Answer from the drawing. Dimensions are ordinates in mm from the lowest x, y and z of the part. A direction names the side the tool comes from. Give positions to 0.01 mm unless a question says otherwise; leave off trailing zeros. Order: outer loops, then holes, each group sorted by start corner. A loop starts at its lowest first (then second) coordinate and runs counter-clockwise, first axis right, second up.
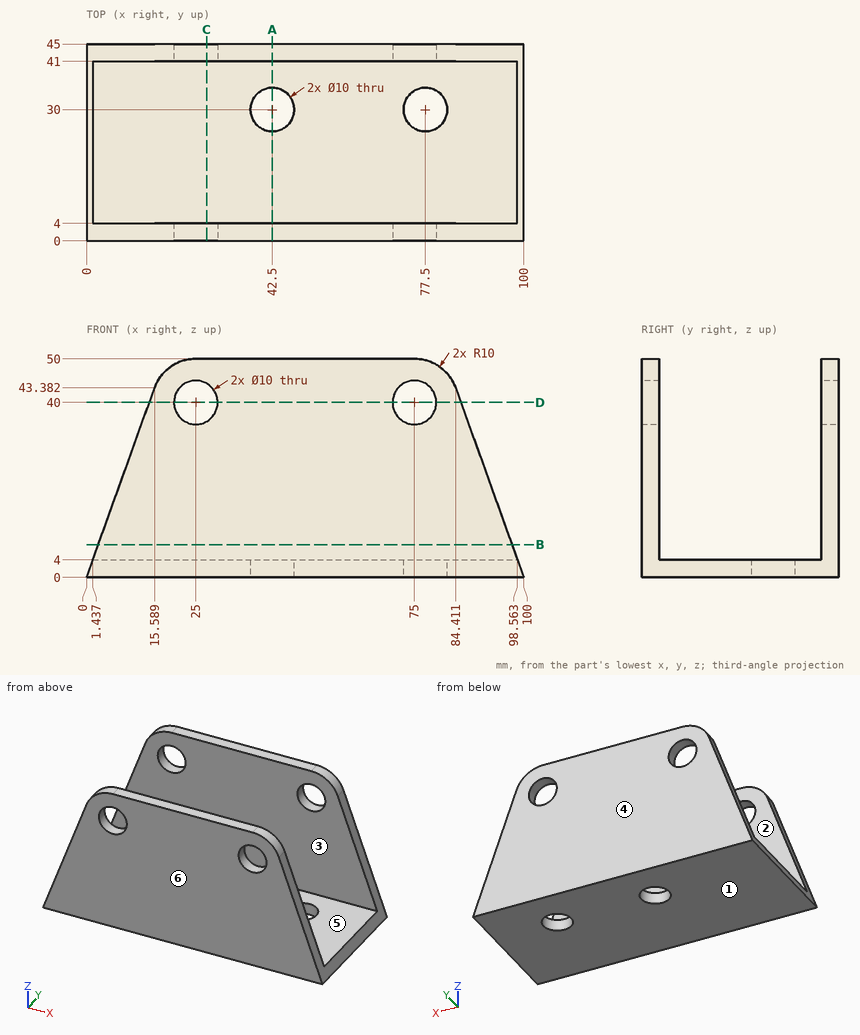
1. Which of the six approach directions +Z, -Z, +X, -X, +Y, -Y give full straight-line access (tool end or side, diameter ignored) to the marked faces 1 and 2?
Findings below:
face 1: -Z, +X, -X, +Y, -Y
face 2: +Z, +X, -X
2. The mould has two halves that part along Y. Classify the marked faces 3, 4, 5 and 6: pulls with the +Y half, pulls with the -Y half, needs draft (parallel to the pull), parting line crosses it, or undercut.
Findings below:
face 3: undercut
face 4: pulls with the +Y half
face 5: undercut
face 6: pulls with the -Y half
3. The part is cut by section A-A (x = 42.5). Write down the section's boundary in (y, z).
Findings below:
outline: (0, 0) - (25, 0) - (25, 4) - (4, 4) - (4, 50) - (0, 50) - close; (35, 0) - (45, 0) - (45, 50) - (41, 50) - (41, 4) - (35, 4) - close
4. The part is cut by section B-B (z = 7.5). Write down the section's boundary in (x, y) (1 decimal).
Findings below:
outline: (2.7, 0) - (97.3, 0) - (97.3, 4) - (2.7, 4) - close; (2.7, 41) - (97.3, 41) - (97.3, 45) - (2.7, 45) - close
5. The part is cut by section C-C (x = 27.5). Write down the section's boundary in (y, z), then the cut area to 3 significant figures.
Findings below:
outline: (0, 0) - (45, 0) - (45, 35.67) - (41, 35.67) - (41, 4) - (4, 4) - (4, 35.67) - (0, 35.67) - close; (0, 44.33) - (4, 44.33) - (4, 50) - (0, 50) - close; (41, 44.33) - (45, 44.33) - (45, 50) - (41, 50) - close
area: 479 mm2
6. Given P1, Ø8, axis at y = 36, z = 19.5, coming from the +X side; P2, Ø8, axis at y = 32.5, z = 6, coming from the +X side; P3, Ø3, axis at y = 5, z = 17, coming from the +X side; P4, Ø18.5, axis at x = 44.5, y = 21, coming from the +Z side, each flat-ended and moving along its own axis, determine where each tip first touches the part or whether it passes through.
Findings below:
P1: passes through
P2: stops at x = 99.28
P3: stops at x = 94.29
P4: stops at z = 4
7. The part is cut by section D-D (z = 40). Write down the section's boundary in (x, y).
Findings below:
outline: (14.37, 0) - (20, 0) - (20, 4) - (14.37, 4) - close; (14.37, 41) - (20, 41) - (20, 45) - (14.37, 45) - close; (30, 0) - (70, 0) - (70, 4) - (30, 4) - close; (30, 41) - (70, 41) - (70, 45) - (30, 45) - close; (80, 0) - (85.63, 0) - (85.63, 4) - (80, 4) - close; (80, 41) - (85.63, 41) - (85.63, 45) - (80, 45) - close
8. Straight lines are drawn through the part: probe 1 along Y at (x, z) = (21, 6); probe 2 along X at (y, z) = (1.1, 40) (1 decimal); probe 3 along Z at (x, y) = (37, 28). For each, find the intervals that lie inside material, in ascending order.
Findings below:
probe 1: y = 0 to 4, 41 to 45
probe 2: x = 14.4 to 20, 30 to 70, 80 to 85.6
probe 3: z = 0 to 4
